```python
from build123d import *

# Parameters (mm, degrees)
SKETCH_1_R          = 2.5
EXTRUDE_1_DEPTH     = 3
SKETCH_4_R          = 5
SKETCH_4_R_2        = 2.5
SKETCH_5_R          = 1.65
CUT_EXTRUDE_1_DEPTH = 4
FILLET_1_R          = 1


with BuildPart() as part:
    # Sketch 1 → Extrude 1 (new body)
    with BuildSketch(Plane.XY):
        with BuildLine():
            Line((0, 5), (15, 5))
            ThreePointArc((15, 5), (20, 0), (15, -5))
            Line((15, -5), (0, -5))
            ThreePointArc((0, -5), (-5, 0), (0, 5))
        make_face()
        Circle(SKETCH_1_R, mode=Mode.SUBTRACT)
    extrude(amount=-EXTRUDE_1_DEPTH)

    # Sweep 1: sweep along a path in Sketch 6
    with BuildLine(Plane(origin=(0, 0, 0), x_dir=(0, 0, 1), z_dir=(0.64278761, 0.766044443, 0))) as sweep_1_path:
        ThreePointArc((0, 0), (5, 1.339745962), (8.660254038, 5))
    # Sketch 4 → Sweep 1 (sweep)
    with BuildSketch(Plane.XY):
        Circle(SKETCH_4_R)
        Circle(SKETCH_4_R_2, mode=Mode.SUBTRACT)
    sweep(path=sweep_1_path.line)

    # Sketch 5 → Cut-Extrude 1 (cut, through all)
    with BuildSketch(Plane.XY):
        with Locations((8, 0)):
            Circle(SKETCH_5_R)
        with Locations((15, 0)):
            Circle(SKETCH_5_R)
    extrude(amount=-CUT_EXTRUDE_1_DEPTH, mode=Mode.SUBTRACT)

    # Fillet 1
    fillet_1_edges = [part.edges().sort_by_distance(p)[0] for p in [
        (2.063752327, -3.829442894, 10.318788908),
    ]]
    fillet(fillet_1_edges, radius=FILLET_1_R)


solid = part.part
```
Geometry check sheet. Reference: the model listing, model coordinates, mm. A direction names the side the tool comes from. Coordinates: 2 decimals unless noted, no trailing zeros. Loops run counter-clockwise (first coordinate to the right, second up) from the corner with the lowest first, then second, coordinate; pieces in that order, holes last. Notation, with made-up numbers: (31.25, 81.25) - (89.25, 81.25) arc R15 ccw to (89.25, 87.25) - close; hole circle Ø6 at (9, -31.75). An arc over 180 degrees is marked (long way). One line per item, written item: value. Start each with the question number.
(1) Cross-section at B-B on z = -1. Enter the section's corners in (x, y).
(2) Cross-section at A-A on x = 8. Enter the section's corners in (y, z).
(3) Mould release check, pull along Y, two halves, no side actions. Record for faces 6 (the flat face through (7, 5, -1)), 7 (the flat face through (8, -2, -3)), 8 (the cylindrical face through (-0.54, -2.44, -1.48)): released by +Y, released by -Y, zero draft, split by the parting line, or undercut.
(4) Depth check by flat-ended pin: P1, Ø4, axis at x = 11, z = 0.5, coming from the -Y side; P2, Ø3, axis at x = 15, y = 0, coming from the +Z side; P3, Ø2, axis at y = 2, z = 9.5, coming from the +X side; P4, Ø1, axis at y = 2, z = 1.5, coming from the -X side. Enter the tip coordinate at first touch or a pass-through.
(5) Material ranges on line 1 (Y direction, x = 8, z = -1.4); line 2 (Y direction, x = -0.5, z = 3); line 3 (Z direction, x = 8.5, y = -2.5), recorded low to high. Write a range as [from, to].
(6) Cross-section at C-C on y = 0. Count the separate pieces of the cut face and the enclosed holes in it, plus the area to 3 significant figures.
(7) Tool access check on faces 1 (the cylindrical face through (-5, 0, -1)), 2 (the flat face through (8, -5, -1)), 3 (the flat face through (6.5, -2.6, 5.8)), 4 (the cylindrical face through (6.784, 1.115, -1.479)), 5 (the cylindrical face through (16.574, 0.496, -1.479)). Record the directions out of +Z, -Z, +X, -X, +Y, -Y that give a thin tool (end or side, any length) a straight path to the whole face; none if there is none.
Results below:
1. outline: (0, -5) - (15, -5) arc R5 ccw to (15, 5) - (0, 5) arc R5 ccw to start; hole circle Ø5 at (0, 0); hole circle Ø3.3 at (8, 0); hole circle Ø3.3 at (15, 0)
2. outline: (-5, -3) - (-1.65, -3) - (-1.65, 0) - (-5, 0) - close; (1.65, -3) - (5, -3) - (5, 0) - (1.65, 0) - close
3. face 6: released by +Y
3. face 7: zero draft
3. face 8: undercut
4. P1: stops at y = -5
4. P2: passes through
4. P3: stops at x = 6.43
4. P4: stops at x = -4.7
5. line 1: y = [-5, -1.65], [1.65, 5]
5. line 2: y = [-5.3, -2.66], [2.13, 4.73]
5. line 3: z = [-3, 0]
6. separate pieces: 3
6. enclosed holes: 0
6. area: 111 mm2
7. face 1: -Z, -X
7. face 2: -Z, +X, -X, -Y
7. face 3: +Z, +X, -Y
7. face 4: -Z
7. face 5: +Z, -Z
